```python
from build123d import *

# Parameters (mm, degrees)
SKETCH1_W             = 8
SKETCH1_H             = 130
BOSS_EXTRUDE1_DEPTH   = 40
SKETCH2_W             = 20.4
SKETCH2_H             = 25
CUT_EXTRUDE1_DEPTH    = 9
FILLET1_R             = 3
SKETCH3_R             = 2.2
CUT_EXTRUDE2_DEPTH    = 41
SKETCH4_R             = 19.5
CUT_EXTRUDE3_DEPTH    = 7.3
CUT_EXTRUDE5_REACH    = 10
SKETCH6_R             = 1.25
CHAMFER1_SIZE         = 3
CHAMFER1_SIZE2        = 2.517298894
CHAMFER1_PART_2_SIZE  = 3
CHAMFER1_PART_2_SIZE2 = 2.517298894


with BuildPart() as part:
    # Sketch1 → Boss-Extrude1 (new body)
    with BuildSketch(Plane.XY):
        Rectangle(SKETCH1_W, SKETCH1_H)
    extrude(amount=-BOSS_EXTRUDE1_DEPTH)

    # Sketch2 → Cut-Extrude1 (cut, through all)
    with BuildSketch(Plane(origin=(4, 0, 0), x_dir=(0, 0, -1), z_dir=(1, 0, 0))):
        with Locations((20, 65)):
            Rectangle(SKETCH2_W, SKETCH2_H)
        with Locations((20, -65)):
            Rectangle(SKETCH2_W, SKETCH2_H)
    extrude(amount=-CUT_EXTRUDE1_DEPTH, mode=Mode.SUBTRACT)

    # Fillet1
    fillet1_edges = [part.edges().sort_by_distance(p)[0] for p in [
        (4, 65, -4.9),
        (-4, 65, -4.9),
        (-4, -65, -4.9),
        (4, -65, -4.9),
        (4, -65, -35.1),
        (-4, -65, -35.1),
        (-4, 65, -35.1),
        (4, 65, -35.1),
    ]]
    fillet(fillet1_edges, radius=FILLET1_R)

    # Sketch3 → Cut-Extrude2 (cut, through all)
    with BuildSketch(Plane.XY):
        with Locations((0, 60)):
            Circle(SKETCH3_R)
        with Locations((0, -60)):
            Circle(SKETCH3_R)
    extrude(amount=-CUT_EXTRUDE2_DEPTH, mode=Mode.SUBTRACT)

    # Sketch4 → Cut-Extrude3 (cut)
    with BuildSketch(Plane.XY):
        with Locations((-17, 0)):
            Circle(SKETCH4_R)
    extrude(amount=-CUT_EXTRUDE3_DEPTH, mode=Mode.SUBTRACT)

    # Sketch6 → Cut-Extrude5 (cut, up to next)
    with BuildSketch(Plane.ZY.offset(4), mode=Mode.PRIVATE) as cut_extrude5_sk1:
        with Locations((-29.5, 33.7)):
            Circle(SKETCH6_R)
    cut_extrude5_tool1 = extrude(cut_extrude5_sk1.sketch, amount=-CUT_EXTRUDE5_REACH, mode=Mode.PRIVATE) & part.part
    add(cut_extrude5_tool1.solids().sort_by_distance((-4, 33.7, -29.5))[0], mode=Mode.SUBTRACT)
    # Sketch6 → Cut-Extrude5 (cut, up to next)
    with BuildSketch(Plane.ZY.offset(4), mode=Mode.PRIVATE) as cut_extrude5_sk2:
        with Locations((-29.5, -18.7)):
            Circle(SKETCH6_R)
    cut_extrude5_tool2 = extrude(cut_extrude5_sk2.sketch, amount=-CUT_EXTRUDE5_REACH, mode=Mode.PRIVATE) & part.part
    add(cut_extrude5_tool2.solids().sort_by_distance((-4, -18.7, -29.5))[0], mode=Mode.SUBTRACT)
    # Sketch6 → Cut-Extrude5 (cut, up to next)
    with BuildSketch(Plane.ZY.offset(4), mode=Mode.PRIVATE) as cut_extrude5_sk3:
        with Locations((-14.5, 33.7)):
            Circle(SKETCH6_R)
    cut_extrude5_tool3 = extrude(cut_extrude5_sk3.sketch, amount=-CUT_EXTRUDE5_REACH, mode=Mode.PRIVATE) & part.part
    add(cut_extrude5_tool3.solids().sort_by_distance((-4, 33.7, -14.5))[0], mode=Mode.SUBTRACT)
    # Sketch6 → Cut-Extrude5 (cut, up to next)
    with BuildSketch(Plane.ZY.offset(4), mode=Mode.PRIVATE) as cut_extrude5_sk4:
        with Locations((-14.5, -18.7)):
            Circle(SKETCH6_R)
    cut_extrude5_tool4 = extrude(cut_extrude5_sk4.sketch, amount=-CUT_EXTRUDE5_REACH, mode=Mode.PRIVATE) & part.part
    add(cut_extrude5_tool4.solids().sort_by_distance((-4, -18.7, -14.5))[0], mode=Mode.SUBTRACT)

    # Chamfer1
    chamfer1_edges = [part.edges().sort_by_distance(p)[0] for p in [
        (-4, 52.5, -20),
    ]]
    chamfer1_side = [part.faces().sort_by_distance(p)[0] for p in [
        (0, 52.5, -20),
    ]]
    chamfer(chamfer1_edges, length=CHAMFER1_SIZE, length2=CHAMFER1_SIZE2, reference=chamfer1_side[0])

    # Chamfer1 part 2
    chamfer1_part_2_edges = [part.edges().sort_by_distance(p)[0] for p in [
        (-4, -52.5, -20),
    ]]
    chamfer1_part_2_side = [part.faces().sort_by_distance(p)[0] for p in [
        (0, -52.5, -20),
    ]]
    chamfer(chamfer1_part_2_edges, length=CHAMFER1_PART_2_SIZE, length2=CHAMFER1_PART_2_SIZE2, reference=chamfer1_part_2_side[0])


solid = part.part
```
The model under review builds one solid part; all positions refer to its coordinate system, in mm. A direction names the side the tool comes from. Round coordinates to 2 decimals unless told otherwise and drop trailing zeros. Order: outer loops, then holes, each group sorted by start corner. A loop starts at its lowest first (then second) coordinate and runs counter-clockwise, first axis right, second up. Notation, with made-up numbers: (-34.5, 20.5) -> (11.5, 20.5) arc R18 ccw to (11.5, 28.5) -> close; hole circle Ø1 at (66.25, 79.25). An arc over 180 degrees is marked (long way). Use a Markdown table: item, result.
Q1. We need section B-B on z = -14.5. Write out the cut boundary in (x, y).
Values:
| item | result |
|---|---|
| outline | (-4, -49.98) -> (-1, -52.5) -> (4, -52.5) -> (4, -19.95) -> (-4, -19.95) -> close; (-4, -17.45) -> (4, -17.45) -> (4, 32.45) -> (-4, 32.45) -> close; (-4, 34.95) -> (4, 34.95) -> (4, 52.5) -> (-1, 52.5) -> (-4, 49.98) -> close |
Q2. We need section D-D on z = -25.5. Write out the cut boundary in (x, y), then the cut area to 3 significant figures.
Values:
| item | result |
|---|---|
| outline | (-4, -49.98) -> (-1, -52.5) -> (4, -52.5) -> (4, 52.5) -> (-1, 52.5) -> (-4, 49.98) -> close |
| area | 832 mm^2 |
Q3. We need section A-A on y = -60. Write out the cut boundary in (x, z).
Values:
| item | result |
|---|---|
| outline | (-4, -40) -> (-2.2, -40) -> (-2.2, -30.2) -> (-4, -30.2) -> close; (-4, -9.8) -> (-2.2, -9.8) -> (-2.2, 0) -> (-4, 0) -> close; (2.2, -40) -> (4, -40) -> (4, -30.2) -> (2.2, -30.2) -> close; (2.2, -9.8) -> (4, -9.8) -> (4, 0) -> (2.2, 0) -> close |
Q4. Tool access review of faces 4 (the cylindrical face through (2.5, -0.2, -3.6)), 5 (the flat face through (-4, -1, -20)): name each direction out of +Z, -Z, +X, -X, +Y, -Y from which nothing blocks a thin tool from reaching the whole face with its end or side.
Values:
| item | result |
|---|---|
| face 4 | +Z, -X |
| face 5 | +Z, -Z, -X, +Y, -Y |
Q5. We need section C-C on y = 33.7. Write out the cut boundary in (x, z).
Values:
| item | result |
|---|---|
| outline | (-4, -40) -> (4, -40) -> (4, -30.75) -> (-4, -30.75) -> close; (-4, -28.25) -> (4, -28.25) -> (4, -15.75) -> (-4, -15.75) -> close; (-4, -13.25) -> (4, -13.25) -> (4, 0) -> (-4, 0) -> close |
Q6. Clearance check with flat-ended pins moving along their axes: P1, Ø4, axis at x = 3, z = -26.5, coming from the -Y side; P2, Ø2.5, axis at x = 1.5, z = -24.5, coming from the +Y side. State where each tip first meets the part, or that it passes through.
Values:
| item | result |
|---|---|
| P1 | stops at y = -52.5 |
| P2 | stops at y = 52.5 |
Q7. Mouldability with a two-part tool opening along Y and no side actions: class faces 1 (the cylindrical face through (3.1, -64.14, -4.97)), 2 (the flat face through (2, 52.5, -20)), 3 (the cylindrical face through (-0.06, 32.48, -14.77)) as +Y half, -Y half, draft (parallel to the pull), parting line (faces both ways), or undercut.
Values:
| item | result |
|---|---|
| face 1 | -Y half |
| face 2 | +Y half |
| face 3 | undercut |
Q8. For line 1 (Y direction, x = 0, z = -33.5); line 2 (Y direction, x = -0.5, z = -29.5); line 3 (Z direction, x = 0.5, y = 57), list the stretches that pass through material, from the lowest coordinate up.
Values:
| item | result |
|---|---|
| line 1 | y = -65 to -62.2, -57.8 to 57.8, 62.2 to 65 |
| line 2 | y = -52.5 to -19.95, -17.45 to 32.45, 34.95 to 52.5 |
| line 3 | z = -40 to -30.2, -9.8 to 0 |
